from build123d import *
from OCP.BRepFilletAPI import BRepFilletAPI_MakeChamfer

# Parameters (mm, degrees)
SKETCH2_R           = 1.8
BOSS_EXTRUDE1_DEPTH = 10
CHAMFER1_SIZE       = 20
CHAMFER1_SIZE_2     = 16.781992624
BOSS_EXTRUDE3_START = 8
SKETCH4_R           = 1.8
BOSS_EXTRUDE3_DEPTH = 8
CUT_EXTRUDE1_DEPTH  = 8
CHAMFER3_SIZE       = 5
CHAMFER3_SIZE2      = 4.195498156
FILLET1_R           = 2


with BuildPart() as part:
    # Sketch2 → Boss-Extrude1 (new body)
    with BuildSketch(Plane(origin=(0, 0, 0), x_dir=(1, 0, 0), z_dir=(0, 1, 0))):
        Polygon((-11.5, 3), (-5, 3), (-5, 17), (-7.5, 17), (-10.5, 17), (-10.5, 23), (-7.5, 23), (7.5, 23), (10.5, 23), (10.5, 17), (7.5, 17), (5, 17), (5, 3), (11.5, 3), (14.5, 3), (14.5, -3), (11.5, -3), (-11.5, -3), (-14.5, -3), (-14.5, 3), align=None)
        with Locations(Location((-11.5, 0, 0), (0, 0, 270))):
            Circle(SKETCH2_R, mode=Mode.SUBTRACT)
        with Locations(Location((11.5, 0, 0), (0, 0, 270))):
            Circle(SKETCH2_R, mode=Mode.SUBTRACT)
        with Locations(Location((-7.5, 20, 0), (0, 0, 270))):
            Circle(SKETCH2_R, mode=Mode.SUBTRACT)
        with Locations(Location((7.5, 20, 0), (0, 0, 270))):
            Circle(SKETCH2_R, mode=Mode.SUBTRACT)
    extrude(amount=-BOSS_EXTRUDE1_DEPTH)

    # Chamfer1
    # the kernel refuses this chamfer: 20, 16.781992624 mm, written as the material it takes off along each edge
    with BuildSketch(Plane(origin=(62.048122067, -10, -23), x_dir=(0, -0.02493932209023439, 0.9996889667359941), z_dir=(-1, 0, 0))) as chamfer1_piece_1:
        Polygon((CHAMFER1_SIZE * 0.999688966736, CHAMFER1_SIZE * 0.0249393220902), (-CHAMFER1_SIZE_2 * 0.0249393220896, CHAMFER1_SIZE_2 * 0.999688966709), (0, 0), align=None)
    extrude(amount=124.096244134, mode=Mode.SUBTRACT)

    # Sketch4 → Boss-Extrude3 (add)
    with BuildSketch(Plane(origin=(0, 0, 0), x_dir=(1, 0, 0), z_dir=(0, 1, 0)).offset(BOSS_EXTRUDE3_START)):
        Polygon((-7.5, 23), (7.5, 23), (10.5, 23), (10.5, 17), (7.5, 17), (5, 17), (5, 3), (11.5, 3), (14.5, 3), (14.5, -3), (11.5, -3), (-11.5, -3), (-14.5, -3), (-14.5, 3), (-11.5, 3), (-5, 3), (-5, 17), (-7.5, 17), (-10.5, 17), (-10.5, 23), align=None)
        with Locations(Location((-11.5, 0, 0), (0, 0, 270))):
            Circle(SKETCH4_R, mode=Mode.SUBTRACT)
        with Locations(Location((11.5, 0, 0), (0, 0, 270))):
            Circle(SKETCH4_R, mode=Mode.SUBTRACT)
        with Locations(Location((7.5, 20, 0), (0, 0, 270))):
            Circle(SKETCH4_R, mode=Mode.SUBTRACT)
        with Locations(Location((-7.5, 20, 0), (0, 0, 270))):
            Circle(SKETCH4_R, mode=Mode.SUBTRACT)
    extrude(amount=-BOSS_EXTRUDE3_DEPTH)

    # Sketch5 → Cut-Extrude1 (cut)
    with BuildSketch(Plane.XZ.offset(10)):
        Polygon((-8.5, 3), (8.5, 3), (8.5, -3), (8.5, -14.917535926), (5, -14.917535926), (-5, -14.917535926), (-8.5, -14.917535926), (-8.5, -3), align=None)
    extrude(amount=-CUT_EXTRUDE1_DEPTH, mode=Mode.SUBTRACT)

    # Chamfer3: one chamfer whose edges measure the first distance from different faces: ONE call of the kernel's chamfer builder (chamfer() names one face for all edges)
    chamfer3_edges_1 = [part.edges().sort_by_distance(p)[0] for p in [
        (8.5, -2, 0),
    ]]
    chamfer3_side_1 = [part.faces().sort_by_distance(p)[0] for p in [
        (8.5, -6, 0),
    ]]
    chamfer3_edges_2 = [part.edges().sort_by_distance(p)[0] for p in [
        (-8.5, -2, 0),
    ]]
    chamfer3_side_2 = [part.faces().sort_by_distance(p)[0] for p in [
        (-8.5, -6, 0),
    ]]
    chamfer3 = BRepFilletAPI_MakeChamfer(part.part.solid().wrapped)
    for e in chamfer3_edges_1:
        chamfer3.Add(CHAMFER3_SIZE, CHAMFER3_SIZE2, e.wrapped, chamfer3_side_1[0].wrapped)  # the first distance lies on this face
    for e in chamfer3_edges_2:
        chamfer3.Add(CHAMFER3_SIZE, CHAMFER3_SIZE2, e.wrapped, chamfer3_side_2[0].wrapped)  # the first distance lies on this face
    add(Compound.cast(chamfer3.Shape()), mode=Mode.REPLACE)

    # Fillet1
    fillet1_edges = [part.edges().sort_by_distance(p)[0] for p in [
        (-10.5, 4, -23),
        (-10.5, 4, -17),
        (-5, 4, -17),
        (5, 4, -17),
        (10.5, 4, -17),
        (10.5, 4, -23),
        (5, 2.585568787, -3),
        (-5, 2.585568787, -3),
        (-8.5, -8.5, -3),
        (-4.304501844, -2, -4.76701437),
        (4.304501844, -2, -4.76701437),
        (8.5, -8.5, -3),
        (8.5, -8.5, 3),
        (-8.5, -8.5, 3),
        (14.5, -1, -3),
        (14.5, -1, 3),
        (-14.5, -1, 3),
        (-14.5, -1, -3),
    ]]
    fillet(fillet1_edges, radius=FILLET1_R)


solid = part.part
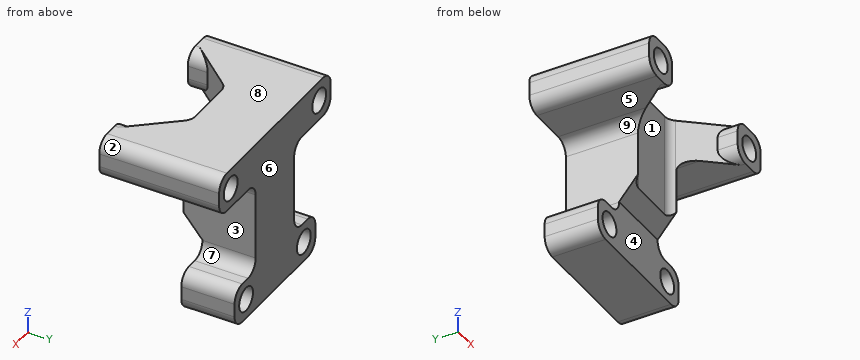
Source: CAD feature listing. Evaluate the final solid. Frame: model axes, mm. Face numbers are marked on the shaded views. A direction names the side the tool comes from. Round coordinates to 2 decimals unless told otherwise and drop trailing zeros. Loops run counter-clockwise (first coordinate to the right, second up) from the corner with the lowest first, then second, coordinate; pieces in that order, holes last. Notation, with made-up numbers: (72.25, 16) -> (94.25, 16) arc R9 ccw to (94.25, 32) -> close; hole circle Ø11 at (-6, 34). An arc over 180 degrees is marked (long way). Answer as a JSON object with one key per item and string values. Group by question number.
Q1. Mould query, pull axis Z, two halves, no side actions, for the marked faces 6, 7, 8 and 9. Classes: pulls with the +Z half, pulls with the -Z half, needs draft (parallel to the pull), parting line crosses it, or undercut.
Q2. Contact query for flat-ended pins moving along their axis: P1, Ø10, axis at x = 0, z = -15.5, coming from the -Y side (3 decimals); P2, Ø6, axis at x = 8.5, y = -5, coming from the -Z side; P3, Ø4, axis at y = 0, z = -16.5, coming from the -X side. Output: stop coordinate, or through.
Q3. Section query D-D (y = -1.5). Output: boundary loops of the cut face in (x, z).
Q4. Section query A-A (x = 11.5). Output: boundary loops of the cut face in (y, z).
Q5. Access query for the marked faces 1, 2, 3, 4 and 5. Directions: +Z, -Z, +X, -X, +Y, -Y. A direction counts if a zero-diameter tool reaches every point of the face in a straight line with its end or side. Return the directions, or none.
Q6. Section query B-B (y = -3.5). Output: boundary loops of the cut face in (x, z).
Q7. Ray query, line 1 (X direction, y = 4.25, z = -20); line 2 (X direction, y = 3, z = 0); line 3 (Y direction, x = 3.25, z = -9.75). Return the intervals inside material, ascending. Write a range as from..to.
Q8. Section query C-C (z = -20). Output: boundary loops of the cut face in (x, y), plus the area to 3 significant figures.
Completed:
{
 "1": {"face 6": "needs draft", "face 7": "undercut", "face 8": "pulls with the +Z half", "face 9": "undercut"},
 "2": {"P1": "y = -2.085", "P2": "z = -3.42", "P3": "x = -10.44"},
 "3": {"outline": "(-14.5, -1) arc R2 ccw to (-12.5, -3) -> (-7, -3) arc R2 cw to (-5, -5) -> (-5, -13.13) -> (5, -13.13) -> (5, -5) arc R2 cw to (7, -3) -> (12.5, -3) arc R2 ccw to (14.5, -1) -> (14.5, 1) arc R2 ccw to (12.5, 3) -> (-12.5, 3) arc R2 ccw to (-14.5, 1) -> close; hole circle Ø3.6 at (-11.5, 0); hole circle Ø3.6 at (11.5, 0)"},
 "4": {"outline": "(-10, -3) -> (8, -3) -> (8, -1.8) -> (-10, -1.8) -> close; (-10, 1.8) -> (8, 1.8) -> (8, 3) -> (-10, 3) -> close"},
 "5": {"face 1": "+Z, -Z, -Y", "face 2": "+Z, +X, +Y, -Y", "face 3": "+X, +Y, -Y", "face 4": "-Z, +X, -X, -Y", "face 5": "-X, +Y, -Y"},
 "6": {"outline": "(-14.5, -1) arc R2 ccw to (-12.5, -3) -> (-7, -3) arc R2 cw to (-5.56, -3.61) -> (-5.56, 3) -> (-12.5, 3) arc R2 ccw to (-14.5, 1) -> close; (5.56, -3.61) arc R2 cw to (7, -3) -> (12.5, -3) arc R2 ccw to (14.5, -1) -> (14.5, 1) arc R2 ccw to (12.5, 3) -> (5.56, 3) -> close; hole circle Ø3.6 at (-11.5, 0); hole circle Ø3.6 at (11.5, 0)"},
 "7": {"line 1": "-10.5..-9.3, -5.7..5.7, 9.3..10.5", "line 2": "-14.5..-13.3, -9.7..9.7, 13.3..14.5", "line 3": "-2..8"},
 "8": {"outline": "(-10.5, 0) -> (-9.3, 0) -> (-9.3, 8) -> (-10.5, 8) -> close; (-5.7, 0) -> (5.7, 0) -> (5.7, 8) -> (-5.7, 8) -> close; (9.3, 0) -> (10.5, 0) -> (10.5, 8) -> (9.3, 8) -> close", "area": "110 mm²"}
}
